from build123d import *

# Parameters (mm, degrees)
F1_DEPTH = 745
F2_W     = 100
F2_H     = 60
F4_W     = 100
F4_H     = 60


with BuildPart() as f1:
    # F0 (on Right) → F1 (new body, symmetric)
    with BuildSketch(Plane.YZ):
        with BuildLine():
            Line((0, -140), (0, 0))
            Line((0, 0), (-95, 0))
            Line((-95, 0), (-95, -10))
            Line((-95, -10), (-200, -40))
            Line((-200, -40), (-200, -140))
            Line((-200, -140), (-190, -140))
            ThreePointArc((-190, -140), (-185, -135), (-180, -140))
            Line((-180, -140), (0, -140))
        make_face()
    extrude(amount=F1_DEPTH, both=True)

    # F2 (on face) → F3 (join, up to the next surface of F1)
    with BuildSketch(Plane.XY):
        with Locations((-695, -125)):
            Rectangle(F2_W, F2_H)
    extrude(until=Until.NEXT, dir=(0, 0, -1))

    # F4 (on face) → F5 (join, up to the next surface of F1)
    with BuildSketch(Plane.XY):
        with Locations((695, -125)):
            Rectangle(F4_W, F4_H)
    extrude(until=Until.NEXT, dir=(0, 0, -1))


solid = f1.part
The listing builds one solid part. Answer for the finished solid, in the listing's coordinates (mm). A direction names the side the tool comes from. Coordinates: 2 decimals unless noted, no trailing zeros. Write each loop counter-clockwise with the first axis right and the second up, starting at its lowest first coordinate (ties: lowest second). Pieces come first, ordered by that corner, then holes. Notation, with made-up numbers: M 72.5,39 L 125.5,39 A35 cw 125.5,76 Z; hole C 18.25,-38 d11. An arc over 180 degrees is marked long. Put each result on its own line as item: value. Start each with the question number.
1. For a pull along X with two mould halves and no side action, classify faces 1 (the flat face through (-645, -132, -10)), 2 (the flat face through (745, -101, -69)), 3 (the flat face through (-10, -59, 0)) as pulls with the +X half, pulls with the -X half, needs draft (parallel to the pull), parting line crosses it, or undercut.
2. Consider line 1 (X direction, y = -134, z = -6.5); line 2 (Z direction, x = 145.5, y = -159.5); line 3 (Y direction, x = -624, z = -7). Determine where each line is inside the solid, lowest interval first. Write a range as from..to.
3. A cutting plane is placed at B-B on y = -138.5. Write down the section's boundary in (x, z), then the cut area to 3 significant figures.
4. A flat-ended cylindrical pin translates along its axis: P1, Ø5, axis at x = 211.5, z = -4.5, coming from the -Y side. Find the tip coordinate at first contact, or state that the pin passes through.
5. A cutting plane is placed at A-A on x = -402. Write down the section's boundary in (y, z), then the cut area to 3 significant figures.
6. Which of the six approach directions +Z, -Z, +X, -X, +Y, -Y give full straight-line access (tool end or side, diameter ignored) to faces 4 (the flat face through (10, -200, -89)), 5 (the flat face through (694, -155, -13)), 6 (the flat face through (645, -132, -10))?
Resolved:
1. face 1: undercut
1. face 2: pulls with the +X half
1. face 3: needs draft
2. line 1: x = -745..-645, 645..745
2. line 2: z = -140..-28.43
2. line 3: y = -95..0
3. outline: M -745,-140 L 745,-140 L 745,0 L 645,0 L 645,-22.43 L -645,-22.43 L -645,0 L -745,0 Z
3. area: 180,000 mm2
4. P1: stops at y = -95
5. outline: M -200,-140 L -190,-140 A5 cw -180,-140 L 0,-140 L 0,0 L -95,0 L -95,-10 L -200,-40 Z
5. area: 25,300 mm2
6. face 4: +Z, -Z, +X, -X, -Y
6. face 5: +Z, +X, -X, -Y
6. face 6: +Z, -Y
